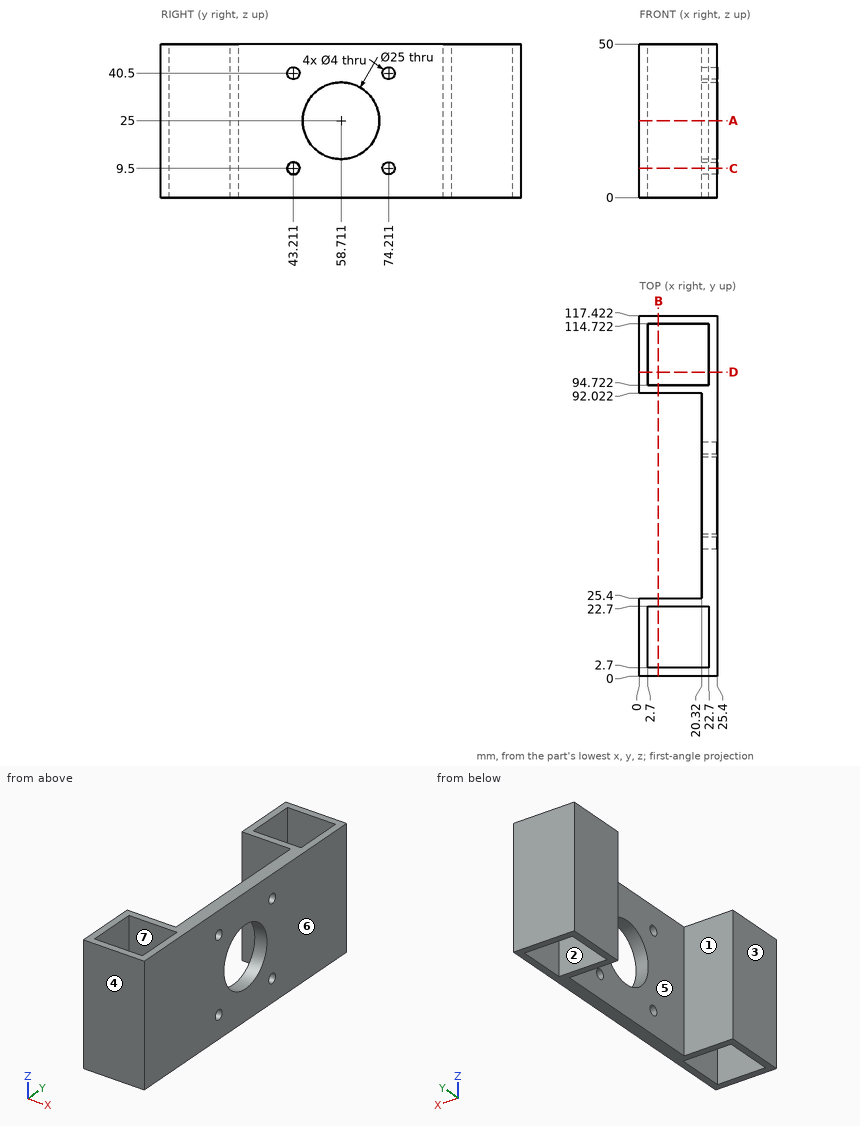
Here's the drawing with two shaded views (mm, measured from the low corner). I have some questions. A direction names the side the tool comes from. Round coordinates to 2 decimals unless told otherwise and drop trailing zeros. Loops run counter-clockwise (first coordinate to the right, second up) from the corner with the lowest first, then second, coordinate; pieces in that order, holes last.
Item 1: Will this pin go through, and if not, where does the flat tip stop? pin 1 Ø15 at (y, z) = (68.5, 31.5) entering from -X.
Item 2: Please list where these lines run through material, in increasing order: L1, parallel to Y at x = 11.5, z = 23; L2, parallel to Y at x = 22.3, z = 9.5; L3, parallel to Y at x = 23.65, z = 9.5.
Item 3: Which directions (+Z, -Z, +X, -X, +Y, -Y) give clear straight access to the entire face, cutting with the end or side of a thin tool? Please do the marked faces 1, 2 and 3.
Item 4: Suppose I cut it at D-D, the plane y = 99. Write out the boundary of the cut face in (x, z).
Item 5: If we mould it in two halves opening along Y, with no side actions, what happens to the marked faces 4, 5, 6 and 7? For each: +Y half, -Y half, draft (parallel to the pull), parting line (faces both ways), or undercut.
Item 6: Suppose I cut it at B-B, the plane x = 6.25. Write out the boundary of the cut face in (y, z).
Item 7: Suppose I cut it at A-A, the plane z = 25. Write out the boundary of the cut face in (x, y).
Item 8: Suppose I cut it at C-C, the plane z = 9.5. Write out the boundary of the cut face in (x, y), then the cut area to 3 significant figures.
Reported:
1. pin 1: stops at x = 20.32
2. L1: y = 0 to 2.7, 22.7 to 25.4, 92.02 to 94.72, 114.72 to 117.42
2. L2: y = 0 to 2.7, 22.7 to 41.21, 45.21 to 72.21, 76.21 to 94.72, 114.72 to 117.42
2. L3: y = 0 to 41.21, 45.21 to 72.21, 76.21 to 117.42
3. face 1: +Z, -Z, -X
3. face 2: +Z, -Z
3. face 3: +Z, -Z, -X, +Y, -Y
4. outline: (0, 0) - (2.7, 0) - (2.7, 50) - (0, 50) - close; (22.7, 0) - (25.4, 0) - (25.4, 50) - (22.7, 50) - close
5. face 4: -Y half
5. face 5: undercut
5. face 6: draft
5. face 7: undercut
6. outline: (0, 0) - (2.7, 0) - (2.7, 50) - (0, 50) - close; (22.7, 0) - (25.4, 0) - (25.4, 50) - (22.7, 50) - close; (92.02, 0) - (94.72, 0) - (94.72, 50) - (92.02, 50) - close; (114.72, 0) - (117.42, 0) - (117.42, 50) - (114.72, 50) - close
7. outline: (0, 0) - (25.4, 0) - (25.4, 46.21) - (20.32, 46.21) - (20.32, 25.4) - (0, 25.4) - close; (0, 92.02) - (20.32, 92.02) - (20.32, 71.21) - (25.4, 71.21) - (25.4, 117.42) - (0, 117.42) - close; hole (2.7, 2.7) - (22.7, 2.7) - (22.7, 22.7) - (2.7, 22.7) - close; hole (2.7, 94.72) - (22.7, 94.72) - (22.7, 114.72) - (2.7, 114.72) - close
8. outline: (0, 0) - (25.4, 0) - (25.4, 41.21) - (20.32, 41.21) - (20.32, 25.4) - (0, 25.4) - close; (0, 92.02) - (20.32, 92.02) - (20.32, 76.21) - (25.4, 76.21) - (25.4, 117.42) - (0, 117.42) - close; (20.32, 45.21) - (25.4, 45.21) - (25.4, 72.21) - (20.32, 72.21) - close; hole (2.7, 2.7) - (22.7, 2.7) - (22.7, 22.7) - (2.7, 22.7) - close; hole (2.7, 94.72) - (22.7, 94.72) - (22.7, 114.72) - (2.7, 114.72) - close
8. area: 788 mm2
